The listing builds one solid part. Answer for the finished solid, in the listing's coordinates (mm). A direction names the side the tool comes from. Coordinates: 2 decimals unless noted, no trailing zeros. Order: outer loops, then holes, each group sorted by start corner. A loop starts at its lowest first (then second) coordinate and runs counter-clockwise, first axis right, second up. Notation, with made-up numbers: (17.5, 10) -> (59.5, 10) arc R18 ccw to (59.5, 45) -> close; hole circle Ø2 at (70.25, -25). An arc over 180 degrees is marked (long way). Write each question's results on one line, items separated by ' | '. Start each with the question number.
(1) The part is cut by section C-C, the plane z = 8.25. Give the vertices of the cut face in (x, y), then the cut area to 3 significant figures.
(2) Straight lines are drawn through the part: L1, parallel to X at y = 4, z = 11; L2, parallel to Z at x = 4.75, y = 16; L3, parallel to Z at x = 7, y = 20.5. For each, find the intervals that lie inside material, in ascending order.
(3) The part is cut by section B-B, the plane y = 19. Give the vertices of the cut face in (x, z).
(4) The part is cut by section D-D, the plane y = 5.5. Give the vertices of the cut face in (x, z).
(5) A tool of negligible diameter and unlimited length cuts with its end or side. For faces 1 (the face through (7.01, 12.65, 11.57)), 2 (the face through (4, 16, 13)), 3 (the face through (4, 16, 0)), from which of +Z, -Z, +X, -X, +Y, -Y can it reach the whole face along a straight path? Write none if from no direction.
(6) Determine the mould class of faces 4 (the face through (1.014, 19.955, 11.61)), 5 (the face through (7, 32.5, 7)), 6 (the face through (8, 16, 8)), 7 (the face through (1.014, 5.705, 6.11)) for opening direction Y: +Y half, -Y half, draft (parallel to the pull), parting line (faces both ways), or undercut.
(7) The part is cut by section A-A, the plane x = 3.25. Give the vertices of the cut face in (y, z), then the cut area to 3 significant figures.
(8) Given pin 1 (1.6 mm diameter, centred on x = 0.5, z = 6.5, fed in from -Y), flat-ended and moving along its own axis, determine where the tip first touches the part or whether it passes through.
```python
from build123d import *

# Parameters (mm, degrees)
SKETCH1_W           = 8
SKETCH1_H           = 15
SKETCH1_W_2         = 4
SKETCH1_H_2         = 11
BOSS_EXTRUDE1_DEPTH = 32.5
CUT_EXTRUDE1_DEPTH  = 37.67764987


with BuildPart() as part:
    # Sketch1 → Boss-Extrude1 (new body)
    with BuildSketch(Plane(origin=(0, 0, 0), x_dir=(1, 0, 0), z_dir=(0, 1, 0))):
        with Locations((4, -7.5)):
            Rectangle(SKETCH1_W, SKETCH1_H)
        with Locations((4, -7.5)):
            Rectangle(SKETCH1_W_2, SKETCH1_H_2, mode=Mode.SUBTRACT)
    extrude(amount=BOSS_EXTRUDE1_DEPTH)

    # Sketch2 → Cut-Extrude1 (cut, through all)
    with BuildSketch(Plane(origin=(8, 0, 0), x_dir=(0, 0, -1), z_dir=(1, 0, 0))):
        Polygon((-10.320250812, 30.5), (-4.679749188, 30.5), (-7.5, 23.192986532), align=None)
        Polygon((-13, 23.557013468), (-10.179749188, 16.25), (-13, 8.942986532), align=None)
        Polygon((-2, 23.557013468), (-4.820250812, 16.25), (-2, 8.942986532), align=None)
        Polygon((-7.5, 9.307013468), (-4.679749188, 2), (-10.320250812, 2), align=None)
    extrude(amount=-CUT_EXTRUDE1_DEPTH, mode=Mode.SUBTRACT)


solid = part.part
```
Established:
1) outline: (0, 0) -> (2, 0) -> (2, 2) -> (0, 2) -> close; (0, 7.36) -> (2, 7.36) -> (2, 25.14) -> (0, 25.14) -> close; (0, 30.5) -> (2, 30.5) -> (2, 32.5) -> (0, 32.5) -> close; (6, 0) -> (8, 0) -> (8, 2) -> (6, 2) -> close; (6, 7.36) -> (8, 7.36) -> (8, 25.14) -> (6, 25.14) -> close; (6, 30.5) -> (8, 30.5) -> (8, 32.5) -> (6, 32.5) -> close | area: 87.1 mm^2
2) L1: x = 0 to 2, 6 to 8 | L2: z = 0 to 2, 13 to 15 | L3: z = 0 to 2, 3.18 to 11.82, 13 to 15
3) outline: (0, 0) -> (8, 0) -> (8, 2) -> (0, 2) -> close; (0, 3.76) -> (2, 3.76) -> (2, 11.24) -> (0, 11.24) -> close; (0, 13) -> (8, 13) -> (8, 15) -> (0, 15) -> close; (6, 3.76) -> (8, 3.76) -> (8, 11.24) -> (6, 11.24) -> close
4) outline: (0, 0) -> (8, 0) -> (8, 6.03) -> (6, 6.03) -> (6, 2) -> (2, 2) -> (2, 6.03) -> (0, 6.03) -> close; (0, 8.97) -> (2, 8.97) -> (2, 13) -> (6, 13) -> (6, 8.97) -> (8, 8.97) -> (8, 15) -> (0, 15) -> close
5) face 1: +X, -X | face 2: none | face 3: -Z, +X, -X, +Y, -Y
6) face 4: undercut | face 5: +Y half | face 6: draft | face 7: undercut
7) outline: (0, 0) -> (32.5, 0) -> (32.5, 2) -> (0, 2) -> close; (0, 13) -> (32.5, 13) -> (32.5, 15) -> (0, 15) -> close | area: 130 mm^2
8) pin 1: stops at y = 0
